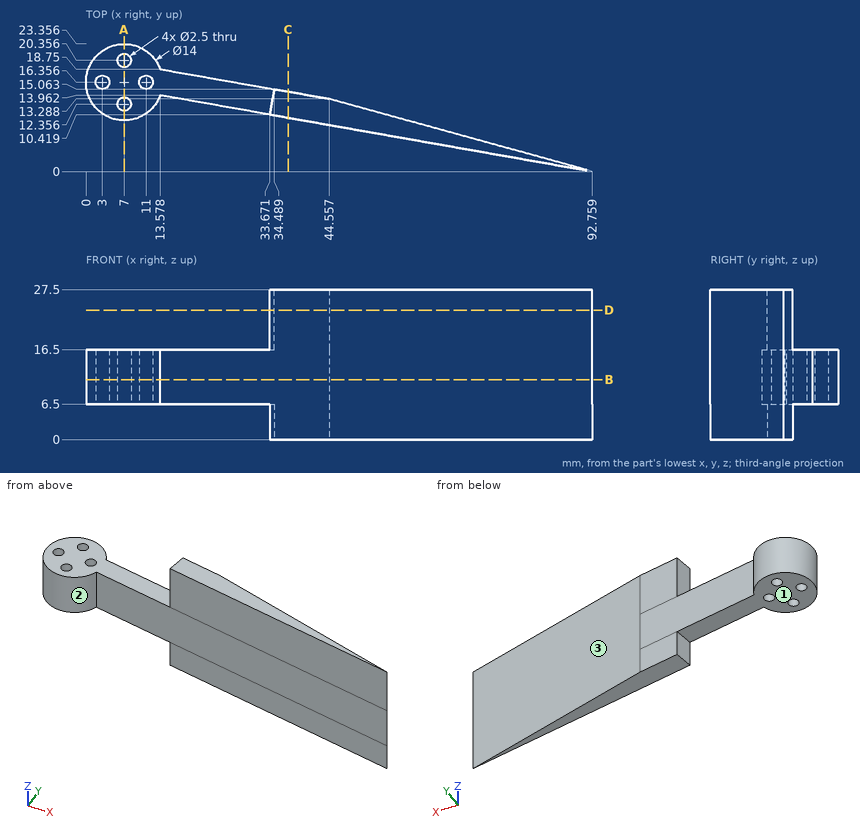
Input: dimensioned drawing with shaded views. Units: mm. Origin: part minimum x, y, z. Give positions to 0.01 mm unless a question says otherwise; leave off trailing zeros. Order: outer loops, then holes, each group sorted by start corner. A loop starts at its lowest first (then second) coordinate and runs counter-clockwise, first axis right, second up.
(1) Material intervals for line 1 along Y through (x, z) = (7, 10) (1 decimal); line 2 along Z through (x, y) = (9.5, 19); line 3 along X through (y, z) = (19.5, 10.25) (1 decimal), sorted ascending.
(2) Section query C-C (x = 37). Return the cut outline in (y, z), plus the area to 3 significant figures.
(3) Pull-direction query (X, two-part tool) for the marked faces 1, 2 and 3; classes: +X half, -X half, draft (parallel to the pull), parting line (faces both ways), or undercut.
(4) Section query A-A (x = 7). Return the cut outline in (y, z) (1 decimal).
(5) Section query D-D (z = 23.75). Return the cut outline in (x, y).
(6) Section query B-B (z = 11). State how many separate pieces and enclosed holes the cut face has.
(7) Contact query for flat-ended pins moving along their axis: P1, Ø3, axis at x = 7, y = 12.36, coming from the -Z side; P2, Ø4, axis at x = 19.5, y = 16, coming from the +Z side; P3, Ø8, axis at x = 19, z = 20, coming from the +Y side (1 decimal). Output: stop coordinate, or through.
Outcome:
1. line 1: y = 9.4 to 11.1, 13.6 to 19.1, 21.6 to 23.4
1. line 2: z = 6.5 to 16.5
1. line 3: x = 0.7 to 6.1, 7.9 to 13.3
2. outline: (9.83, 0) - (14.62, 0) - (14.62, 27.5) - (9.83, 27.5) - close
2. area: 132 mm2
3. face 1: draft
3. face 2: undercut
3. face 3: +X half
4. outline: (9.4, 6.5) - (11.1, 6.5) - (11.1, 16.5) - (9.4, 16.5) - close; (13.6, 6.5) - (19.1, 6.5) - (19.1, 16.5) - (13.6, 16.5) - close; (21.6, 6.5) - (23.4, 6.5) - (23.4, 16.5) - (21.6, 16.5) - close
5. outline: (33.67, 10.42) - (92.76, 0) - (44.56, 13.29) - (34.49, 15.06) - close
6. separate pieces: 1
6. enclosed holes: 4
7. P1: stops at z = 6.5
7. P2: stops at z = 16.5
7. P3: stops at y = 18.1
